Check sheet for the modelled part. Datum: model origin and axes. Units: mm. A direction names the side the tool comes from. Coordinates: 2 decimals unless noted, no trailing zeros. Loops run counter-clockwise (first coordinate to the right, second up) from the corner with the lowest first, then second, coordinate; pieces in that order, holes last. Notation, with made-up numbers: M 8,43 L 34,43 A23 ccw 34,51 Z; hole C 72.5,4.25 d8. An arc over 180 degrees is marked long. Return JSON: item names as keys, results as strings.
from build123d import *

# Parameters (mm, degrees)
SKETCH1_W           = 50
SKETCH1_H           = 51
BOSS_EXTRUDE1_DEPTH = 2
SKETCH2_R           = 11.05
SKETCH2_R_2         = 1.75
CUT_EXTRUDE1_DEPTH  = 3
SKETCH4_W           = 50
SKETCH4_H           = 2
BOSS_EXTRUDE2_DEPTH = 49
BOSS_EXTRUDE3_DEPTH = 2
BOSS_EXTRUDE4_DEPTH = 2
SKETCH7_R           = 2.55
CUT_EXTRUDE2_DEPTH  = 2
FILLET1_R           = 2
SKETCH8_R           = 2.55
CUT_EXTRUDE4_DEPTH  = 2


with BuildPart() as part:
    # Sketch1 → Boss-Extrude1 (new body)
    with BuildSketch(Plane(origin=(0, 0, 0), x_dir=(1, 0, 0), z_dir=(0, 1, 0))):
        with Locations((0, -4.5)):
            Rectangle(SKETCH1_W, SKETCH1_H)
    extrude(amount=BOSS_EXTRUDE1_DEPTH)

    # Sketch2 → Cut-Extrude1 (cut)
    with BuildSketch(Plane(origin=(0, 2, 0), x_dir=(1, 0, 0), z_dir=(0, 1, 0))):
        with Locations(Location((0, 0, 0), (0, 0, 270))):
            Circle(SKETCH2_R)
        with Locations(Location((-15.5, 15.5, 0), (0, 0, 270))):
            Circle(SKETCH2_R_2)
        with Locations(Location((-15.5, -15.5, 0), (0, 0, 270))):
            Circle(SKETCH2_R_2)
        with Locations(Location((15.5, -15.5, 0), (0, 0, 270))):
            Circle(SKETCH2_R_2)
        with Locations(Location((15.5, 15.5, 0), (0, 0, 270))):
            Circle(SKETCH2_R_2)
    extrude(amount=-CUT_EXTRUDE1_DEPTH, mode=Mode.SUBTRACT)

    # Sketch4 → Boss-Extrude2 (add)
    with BuildSketch(Plane(origin=(0, 2, 0), x_dir=(1, 0, 0), z_dir=(0, 1, 0))):
        with Locations((0, -29)):
            Rectangle(SKETCH4_W, SKETCH4_H)
    extrude(amount=BOSS_EXTRUDE2_DEPTH)

    # Sketch5 → Boss-Extrude3 (add)
    with BuildSketch(Plane(origin=(25, 0, 0), x_dir=(0, 0, -1), z_dir=(1, 0, 0))):
        Polygon((-28, 26.5), (-3.5, 2), (-28, 2), align=None)
    extrude(amount=-BOSS_EXTRUDE3_DEPTH)

    # Sketch6 → Boss-Extrude4 (add)
    with BuildSketch(Plane.ZY.offset(25)):
        Polygon((28, 26.5), (3.5, 2), (28, 2), align=None)
    extrude(amount=-BOSS_EXTRUDE4_DEPTH)

    # Sketch7 → Cut-Extrude2 (cut)
    with BuildSketch(Plane(origin=(0, 0, 28), x_dir=(-1, 0, 0), z_dir=(0, 0, -1))):
        with Locations((0, 22.8)):
            Circle(SKETCH7_R)
        with Locations((0, 42.8)):
            Circle(SKETCH7_R)
        with Locations((15.25, 22.8)):
            Circle(SKETCH7_R)
        with Locations((15.25, 42.8)):
            Circle(SKETCH7_R)
        with Locations(Location((-15.25, 42.8, 0), (0, 0, 180))):
            Circle(SKETCH7_R)
        with Locations(Location((-15.25, 22.8, 0), (0, 0, 180))):
            Circle(SKETCH7_R)
    extrude(amount=-CUT_EXTRUDE2_DEPTH, mode=Mode.SUBTRACT)

    # Fillet1
    fillet1_edges = [part.edges().sort_by_distance(p)[0] for p in [
        (0, 0, 30),
        (0, 2, 28),
    ]]
    fillet(fillet1_edges, radius=FILLET1_R)

    # Sketch8 → Cut-Extrude4 (cut)
    # profile 1 of 2: a face of its own
    with BuildSketch(Plane(origin=(0, 0, 28), x_dir=(-1, 0, 0), z_dir=(0, 0, -1))):
        Polygon((25, 51), (5, 51), (25, 26.5), align=None)
        with Locations((15.25, 42.8)):
            Circle(SKETCH8_R, mode=Mode.SUBTRACT)
    # profile 2 of 2: a face of its own
    with BuildSketch(Plane(origin=(0, 0, 28), x_dir=(-1, 0, 0), z_dir=(0, 0, -1))):
        Polygon((-25, 26.5), (-5, 51), (-25, 51), align=None)
        with Locations((-15.25, 42.8)):
            Circle(SKETCH8_R, mode=Mode.SUBTRACT)
    extrude(amount=-CUT_EXTRUDE4_DEPTH, mode=Mode.SUBTRACT)


solid = part.part
1) Draft check along X on faces 1 (the face through (23, 9, 21)), 2 (the face through (25, 9, 18)), 3 (the face through (0, 27, 28)), 4 (the face through (0.35, 0.57, 29.4)). Enter one of: +X half, -X half, draft (parallel to the pull), parting line (faces both ways), or undercut.
Answers:
{"face 1": "undercut", "face 2": "+X half", "face 3": "undercut", "face 4": "draft"}
2) Section check C-C on x = -15.5. Record the cut outline in (y, z), then the cut area to 3 significant figures.
Answers:
{"outline": "M 0,-21 L 2,-21 L 2,-17.25 L 0,-17.25 Z; M 0,-13.75 L 2,-13.75 L 2,13.75 L 0,13.75 Z; M 0,17.25 L 2,17.25 L 2,26 A2 cw 4,28 L 20.26,28 L 20.26,30 L 2,30 A2 ccw 0,28 Z; M 25.34,28 L 38.14,28 L 38.14,30 L 25.34,30 Z", "area": "150 mm²"}
3) Scan lines: line 1 along X through (y, z) = (1.2, 15.5); line 2 along Y through (x, z) = (0, 29.2); line 3 along X through (y, z) = (20, 22). Record each from-to range of solid material in increasing order. Write a range as [from, to].
Answers:
{"line 1": "[-25, -17.25], [-13.75, 13.75], [17.25, 25]", "line 2": "[0.4, 20.25], [25.35, 40.25], [45.35, 51]", "line 3": "[-25, -23], [23, 25]"}
4) Set-up check for faces 5 (the face through (24, 14.4, 15.9)), 6 (the face through (-23, 9, 21)): record each of +Z, -Z, +X, -X, +Y, -Y from which the full face is reachable in a straight line by a thin tool's end or side.
Answers:
{"face 5": "-Z, +X, -X, +Y", "face 6": "-Z, +Y"}
5) Go/stop test with flat-tipped pins: pin 1 Ø3 at (x, y) = (15, 24) entering from -Z; pin 2 Ø14 at (x, z) = (12, 3.5) entering from +Y; pin 3 Ø4.5 at (x, y) = (-15.25, 22.8) entering from -Z. Record where each tip stops, or that it passes through.
Answers:
{"pin 1": "z = 28", "pin 2": "y = 2", "pin 3": "through"}
6) Section check A-A on y = 22.8. Record the cut outline in (x, z).
Answers:
{"outline": "M -25,24.3 L -23,24.3 L -23,28 L -17.8,28 L -17.8,30 L -25,30 Z; M -12.7,28 L -2.55,28 L -2.55,30 L -12.7,30 Z; M 2.55,28 L 12.7,28 L 12.7,30 L 2.55,30 Z; M 17.8,28 L 23,28 L 23,24.3 L 25,24.3 L 25,30 L 17.8,30 Z"}
7) Section check B-B on z = 15.5. Record the cut outline in (x, y).
Answers:
{"outline": "M -25,0 L -17.25,0 L -17.25,2 L -23,2 L -23,14 L -25,14 Z; M -13.75,0 L 13.75,0 L 13.75,2 L -13.75,2 Z; M 17.25,0 L 25,0 L 25,14 L 23,14 L 23,2 L 17.25,2 Z"}
8) Section check D-D on z = 21.5. Record the cut outline in (x, y), then the cut area to 3 significant figures.
Answers:
{"outline": "M -25,0 L 25,0 L 25,20 L 23,20 L 23,2 L -23,2 L -23,20 L -25,20 Z", "area": "172 mm²"}
